Autodesk Inventor part; units mm, degrees
ref_plane "YZ Plane" through (0, 0, 0) normal (1, 0, 0) x (0, 1, 0)
ref_plane "XZ Plane" through (0, 0, 0) normal (0, 1, 0) x (-1, 0, 0)
ref_plane "XY Plane" through (0, 0, 0) normal (0, 0, 1) x (1, 0, 0)
sketch "Boceto1" plane through (0, 0, 0) normal (0, 1, 0) x (-1, 0, 0)
  line L0 (0, 0) -> (100, 0)
  line L1 (100, 0) -> (100, -100)
  line L2 (100, -100) -> (0, -100)
  line L3 (0, -100) -> (0, 0)
  line L4 (100, 0) -> (65, 0)
  line L5 (65, 0) -> (65, -50)
  line L6 (65, -100) -> (100, -100)
  line L7 (100, -100) -> (100, 0)
  line L8 (65, -50) -> (100, -50)
  line L9 (65, -50) -> (65, -100)
  line L10 (65, -25) -> (100, -25)
  line L11 (65, -75) -> (100, -75)
  line L12 (103, -103) -> (103, 3)
  line L13 (103, 3) -> (-3, 3)
  line L14 (-3, 3) -> (-3, -103)
  line L15 (-3, -103) -> (103, -103)
  line L16 (65, -72) -> (100, -72)
  line L17 (65, -47) -> (100, -47)
  line L18 (65, -22) -> (100, -22)
  line L19 (62, 0) -> (62, -100)
  dimension "d0" = 100
  dimension "d1" = 100
  dimension "d2" = 3
  dimension "d3" = 3
  dimension "d4" = 3
  dimension "d5" = 3
  dimension "d6" = 3
  dimension "d7" = 35
extrude "Extrusión1" add sketch "Boceto1" along normal blind 20 contours L0 L5 L9 L2 L19 | L18 L1 L10 L5 | L9 L16 L1 L11 | L17 L1 L8 L5 | L15 L14 L13 L12
extrude "Extrusión2" add sketch "Boceto1" against normal blind 3 contours L0 L19 L2 L3 | L0 L5 L9 L2 L19 | L0 L1 L18 L5 | L18 L1 L10 L5 | L9 L11 L1 L2 | L10 L1 L17 L5 | L9 L16 L1 L11 | L17 L1 L8 L5 | L9 L8 L1 L16 | L15 L14 L13 L12
equation "\"d3\" = d2"
equation "\"d4\" = d3"
equation "\"d5\" = d2"
properties part number "Cajita Organizadora"
Could you check a few things on this model? Use its own coordinates, in mm. A direction names the side the tool comes from. Give positions to 0.01 mm unless a question says otherwise; leave off trailing zeros. Write each loop counter-clockwise with the first axis right and the second up, starting at its lowest first coordinate (ties: lowest second). Pieces come first, ordered by that corner, then holes. Notation, with made-up numbers: (46, 72.5) -> (99, 72.5) arc R34 cw to (99, 103.5) -> close; hole circle Ø4 at (-20, 9). An arc over 180 degrees is marked (long way). Write each question's results on one line, items separated by ' | '.
1. I want a section at C-C, the plane z = -9.5. Write out the boundary of the cut face in (x, y), then the cut area to 3 significant figures.
Check sheet entries:
outline: (-103, -3) -> (3, -3) -> (3, 20) -> (0, 20) -> (0, 0) -> (-62, 0) -> (-62, 20) -> (-65, 20) -> (-65, 0) -> (-100, 0) -> (-100, 20) -> (-103, 20) -> close | area: 498 mm²
2. I want a section at D-D, the plane x = -26. Write out the boundary of the cut face in (y, z).
Check sheet entries:
outline: (-3, -103) -> (20, -103) -> (20, -100) -> (0, -100) -> (0, 0) -> (20, 0) -> (20, 3) -> (-3, 3) -> close
3. I need wall thicknesses on L1, parallel to Z at x = -94.5, y = 15; L2, parallel to X at y = 9.5, z = -85.5; L3, parallel to X at y = 12.25, z = -72.5. Which ranges of each line are inside material? Lowest first, please.
Check sheet entries:
L1: z = -103 to -100, -75 to -72, -50 to -47, -25 to -22, 0 to 3 | L2: x = -103 to -100, -65 to -62, 0 to 3 | L3: x = -103 to -62, 0 to 3
4. If we mould it in two halves opening along Z, with no side actions, what happens to faces 3 (the flat face through (-65, 10, -11)), 4 (the flat face through (-49, 8, -103)), 5 (the flat face through (3, 8, -49))? For each: released by +Z, released by -Z, zero draft, split by the parting line, or undercut.
Check sheet entries:
face 3: undercut | face 4: released by -Z | face 5: zero draft
5. Will this pin go through, and if not, where does the flat tip stop? pin 1 Ø11 at (x, z) = (-91, -11.5) entering from +Y.
Check sheet entries:
pin 1: stops at y = 0
6. I want a section at B-B, the plane y = 2. Write out the boundary of the cut face in (x, z), then the cut area to 3 significant figures.
Check sheet entries:
outline: (-103, -103) -> (3, -103) -> (3, 3) -> (-103, 3) -> close; hole (-100, -100) -> (-65, -100) -> (-65, -75) -> (-100, -75) -> close; hole (-100, -72) -> (-65, -72) -> (-65, -50) -> (-100, -50) -> close; hole (-100, -47) -> (-65, -47) -> (-65, -25) -> (-100, -25) -> close; hole (-100, -22) -> (-65, -22) -> (-65, 0) -> (-100, 0) -> close; hole (-62, -100) -> (0, -100) -> (0, 0) -> (-62, 0) -> close | area: 1,850 mm²
7. On a 3-axis mill with a long thin cutter (end or side, diameter ignored), from which of +Z, -Z, +X, -X, +Y, -Y can I reach the whole of each face in a straight line? I mean faces 1 (the flat face through (-31, 10, -100)), 2 (the flat face through (-49, -3, -49)). Say none if no direction works.
Check sheet entries:
face 1: +Y | face 2: +Z, -Z, +X, -X, -Y
8. I want a section at A-A, the plane x = -84.5. Write out the boundary of the cut face in (y, z).
Check sheet entries:
outline: (-3, -103) -> (20, -103) -> (20, -100) -> (0, -100) -> (0, -75) -> (20, -75) -> (20, -72) -> (0, -72) -> (0, -50) -> (20, -50) -> (20, -47) -> (0, -47) -> (0, -25) -> (20, -25) -> (20, -22) -> (0, -22) -> (0, 0) -> (20, 0) -> (20, 3) -> (-3, 3) -> close
